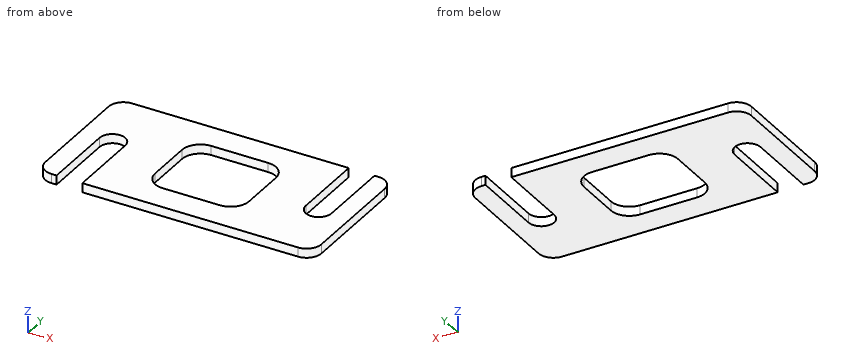
```python
from build123d import *

# Parameters (mm, degrees)
F0_W     = 150
F0_H     = 75
F1_DEPTH = 5
F3_DEPTH = 282
F4_DEPTH = 5.001
F5_W     = 51.0268339871
F5_H     = 45
F6_DEPTH = 5.001
F7_R     = 10
F8_R     = 8


# Not quite as in the source:
# - an extrude ends at something that could not be found from the text; its depth is read off the source's solid


with BuildPart() as f1:
    # F0 (on Top) → F1 (new body)
    with BuildSketch(Plane.XY):
        with Locations((-33.9150866494, -108.2351529738)):
            Rectangle(F0_W, F0_H)
    extrude(amount=F1_DEPTH)

    # F2 (on Top) → F3 (cut, through all)
    with BuildSketch(Plane.XY):
        with BuildLine():
            Line((-98.1348048404, -105.7351529738), (-98.1348048404, -145.7351529738))
            Line((-98.1348048404, -145.7351529738), (-84.1348048404, -145.7351529738))
            Line((-84.1348048404, -145.7351529738), (-84.1348048404, -105.7351529738))
            ThreePointArc((-84.1348048404, -105.7351529738), (-91.1348048404, -98.7351529738), (-98.1348048404, -105.7351529738))
        make_face()
        with BuildLine():
            Line((30.8920291467, -110.7351529738), (30.8920291467, -70.7351529738))
            Line((30.8920291467, -70.7351529738), (16.8920291467, -70.7351529738))
            Line((16.8920291467, -70.7351529738), (16.8920291467, -110.7351529738))
            ThreePointArc((16.8920291467, -110.7351529738), (23.8920291467, -117.7351529738), (30.8920291467, -110.7351529738))
        make_face()
    extrude(amount=-F3_DEPTH, mode=Mode.SUBTRACT)

    # F2 (on Top) → F4 (cut, through all)
    with BuildSketch(Plane.XY):
        with BuildLine():
            Line((-98.1348048404, -105.7351529738), (-98.1348048404, -145.7351529738))
            Line((-98.1348048404, -145.7351529738), (-84.1348048404, -145.7351529738))
            Line((-84.1348048404, -145.7351529738), (-84.1348048404, -105.7351529738))
            ThreePointArc((-84.1348048404, -105.7351529738), (-91.1348048404, -98.7351529738), (-98.1348048404, -105.7351529738))
        make_face()
        with BuildLine():
            Line((30.8920291467, -110.7351529738), (30.8920291467, -70.7351529738))
            Line((30.8920291467, -70.7351529738), (16.8920291467, -70.7351529738))
            Line((16.8920291467, -70.7351529738), (16.8920291467, -110.7351529738))
            ThreePointArc((16.8920291467, -110.7351529738), (23.8920291467, -117.7351529738), (30.8920291467, -110.7351529738))
        make_face()
    extrude(amount=F4_DEPTH, mode=Mode.SUBTRACT)

    # F5 (on face) → F6 (cut, through all)
    with BuildSketch(Plane.XY.offset(5)):
        with Locations((-33.6213878469, -108.2351529738)):
            Rectangle(F5_W, F5_H)
    extrude(amount=-F6_DEPTH, mode=Mode.SUBTRACT)

    # F7
    f7_edges = [f1.edges().sort_by_distance(p)[0] for p in [
        (-8.107971, -85.735153, 2.5),
        (-8.107971, -130.735153, 2.5),
        (-59.134805, -130.735153, 2.5),
        (-59.134805, -85.735153, 2.5),
    ]]
    fillet(f7_edges, radius=F7_R)

    # F8
    f8_edges = [f1.edges().sort_by_distance(p)[0] for p in [
        (41.084913, -145.735153, 2.5),
        (41.084913, -70.735153, 2.5),
        (-108.915087, -70.735153, 2.5),
        (-108.915087, -145.735153, 2.5),
    ]]
    fillet(f8_edges, radius=F8_R)


solid = f1.part
```
Read the model definition and answer for the solid it produces. Units are mm, in the model's axes. Give positions to 0.01 mm unless a question says otherwise; leave off trailing zeros. Loops run counter-clockwise (first coordinate to the right, second up) from the corner with the lowest first, then second, coordinate; pieces in that order, holes last.
Item 1: The part is cut by section D-D (y = -115). Write down the section's boundary in (x, z), and give its area (3 significant figures).
Item 2: The part is cut by section B-B (z = 3). Write down the section's boundary in (x, y), and give its area (3 significant figures).
Item 3: The part is cut by section A-A (y = -81). Write down the section's boundary in (x, z), and give its area (3 significant figures).
Item 4: Find the intervals of material crossed by line 1 along Y through (x, z) = (-34.5, 3.35); line 2 along X through (y, z) = (-110, 2.7); line 3 along X through (y, z) = (-127, 3.1), in increasing order.
Item 5: The part is cut by section C-C (x = -36). Write down the section's boundary in (y, z), and give its area (3 significant figures).
Item 6: This flat-tipped pin is pushed along its axis until it touches: pin 1 Ø8 at (x, y) = (-45.5, -90) entering from -Z. Where does it stop, or does it pass through?
Taken from the geometry:
1. outline: (-108.92, 0) - (-98.13, 0) - (-98.13, 5) - (-108.92, 5) - close; (-84.13, 0) - (-59.13, 0) - (-59.13, 5) - (-84.13, 5) - close; (-8.11, 0) - (18.34, 0) - (18.34, 5) - (-8.11, 5) - close; (29.44, 0) - (41.08, 0) - (41.08, 5) - (29.44, 5) - close
1. area: 369 mm2
2. outline: (-108.92, -137.74) arc R8 ccw to (-100.92, -145.74) - (-98.13, -145.74) - (-98.13, -105.74) arc R7 cw to (-84.13, -105.74) - (-84.13, -145.74) - (33.08, -145.74) arc R8 ccw to (41.08, -137.74) - (41.08, -78.74) arc R8 ccw to (33.08, -70.74) - (30.89, -70.74) - (30.89, -110.74) arc R7 cw to (16.89, -110.74) - (16.89, -70.74) - (-100.92, -70.74) arc R8 ccw to (-108.92, -78.74) - close; hole (-59.13, -120.74) arc R10 ccw to (-49.13, -130.74) - (-18.11, -130.74) arc R10 ccw to (-8.11, -120.74) - (-8.11, -95.74) arc R10 ccw to (-18.11, -85.74) - (-49.13, -85.74) arc R10 ccw to (-59.13, -95.74) - close
2. area: 7,710 mm2
3. outline: (-108.92, 0) - (16.89, 0) - (16.89, 5) - (-108.92, 5) - close; (30.89, 0) - (41.08, 0) - (41.08, 5) - (30.89, 5) - close
3. area: 680 mm2
4. line 1: y = -145.74 to -130.74, -85.74 to -70.74
4. line 2: x = -108.92 to -98.13, -84.13 to -59.13, -8.11 to 16.89, 30.89 to 41.08
4. line 3: x = -108.92 to -98.13, -84.13 to -56.93, -10.31 to 41.08
5. outline: (-145.74, 0) - (-130.74, 0) - (-130.74, 5) - (-145.74, 5) - close; (-85.74, 0) - (-70.74, 0) - (-70.74, 5) - (-85.74, 5) - close
5. area: 150 mm2
6. pin 1: passes through
